Here's the drawing with two shaded views (mm, measured from the low corner). I have some questions. Give positions to 0.01 mm unless a question says otherwise; leave off trailing zeros. Write each loop counter-clockwise with the first axis right and the second up, starting at its lowest first coordinate (ties: lowest second). Pieces come first, ordered by that corner, then holes. Notation, with made-up numbers: (81, 33.5) - (114, 33.5) arc R13 cw to (114, 55.5) - close; hole circle Ø9 at (86.25, 89). An arc over 180 degrees is marked (long way). Write item = value, one per line.
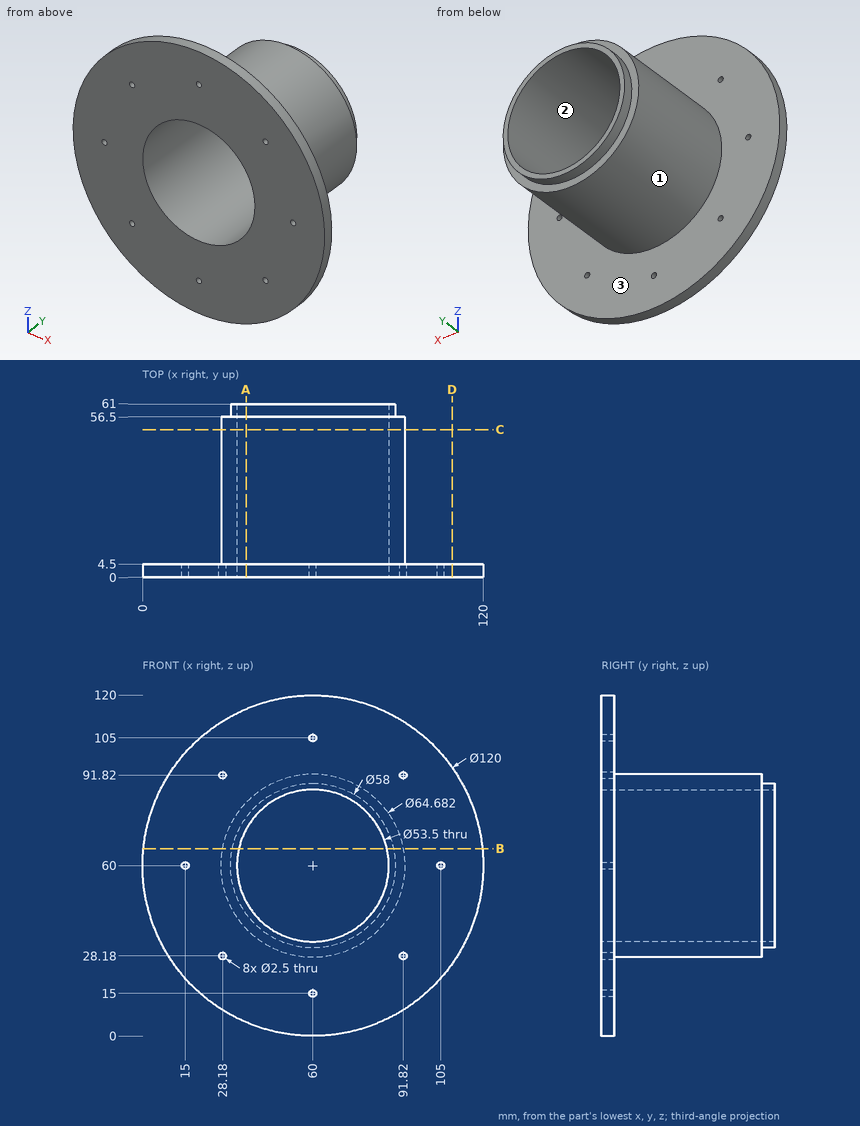
1. If we section it at A-A, the plane x = 36.5: Please give me the cut outline in (y, z).
Filled sheet:
outline = (0, 4.79) - (4.5, 4.79) - (4.5, 37.78) - (56.5, 37.78) - (56.5, 43.01) - (61, 43.01) - (61, 47.22) - (0, 47.22) - close; (0, 72.78) - (61, 72.78) - (61, 76.99) - (56.5, 76.99) - (56.5, 82.22) - (4.5, 82.22) - (4.5, 115.21) - (0, 115.21) - close
2. If we section it at C-C, the plane y = 52: Please give me the cut outline in (x, z), and give its area (3 significant figures).
Filled sheet:
outline = circle Ø64.68 at (60, 60); hole circle Ø53.5 at (60, 60)
area = 1,040 mm2
3. For pin 1 (3 mm diameter, centred on x = 105, z = 60, fed in from +Y); pin 2 (1.5 mm diameter, centred on x = 30, y = 24.5, fed in from -Z); pin 3 (5 mm diameter, centred on y = 35, z = 82.5, fed in from +X) (1 decimal), each with a flat end and sliding along its axis, tell me the tip position at first contact or that it passes through.
Filled sheet:
pin_1 = 4.5
pin_2 = 46.2
pin_3 = 85.4
4. If we section it at B-B, the plane z = 66: Please give me the cut outline in (x, y).
Filled sheet:
outline = (0.3, 0) - (33.93, 0) - (33.93, 61) - (31.63, 61) - (31.63, 56.5) - (28.22, 56.5) - (28.22, 4.5) - (0.3, 4.5) - close; (86.07, 0) - (119.7, 0) - (119.7, 4.5) - (91.78, 4.5) - (91.78, 56.5) - (88.37, 56.5) - (88.37, 61) - (86.07, 61) - close
5. Thinking about a two-plate mould opening in Z: for the marked faces 1, 2 and 3, which applies, pulls with the +Z half, pulls with the -Z half, needs draft (parallel to the pull), parting line crosses it, or undercut?
Filled sheet:
face_1 = parting line crosses it
face_2 = undercut
face_3 = needs draft
6. If we section it at D-D, the plane x = 109: Please give me the cut outline in (y, z).
Filled sheet:
outline = (0, 25.37) - (4.5, 25.37) - (4.5, 94.63) - (0, 94.63) - close
7. I need wall thicknesses on line 1 (X direction, y = 31, z = 60); line 2 (Y direction, x = 17, z = 61); line 3 (X direction, y = 4, z = 43.5) (1 decimal). Which ranges of each line are inside material? Lowest first, please.
Filled sheet:
line_1 = 27.66 to 33.25, 86.75 to 92.34
line_2 = 0 to 4.5
line_3 = 2.3 to 38.9, 81.1 to 117.7
